from build123d import *

# Parameters (mm, degrees)
F1_R     = 7.008857
F1_R_2   = 6.918989
F1_R_3   = 6.910628
F1_R_4   = 85
F1_R_5   = 7.545233
F2_DEPTH = 3


with BuildPart() as f2:
    # F1 (on Top) → F2 (new body)
    with BuildSketch(Plane.XY):
        with BuildLine():
            ThreePointArc((133.07327, 178.290789), (197.066851, 100.910925), (219.991151, 3.14949))
            ThreePointArc((219.991151, 3.14949), (197.066851, -94.611945), (133.07327, -171.991809))
            Line((133.07327, -171.991809), (156.635002, -171.991809))
            ThreePointArc((156.635002, -171.991809), (214.509219, -92.785593), (234.991151, 3.14949))
            ThreePointArc((234.991151, 3.14949), (214.509219, 99.084573), (156.635002, 178.290789))
            Line((156.635002, 178.290789), (133.07327, 178.290789))
        make_face()
        with BuildLine():
            ThreePointArc((-132.922132, -171.991809), (-219.840013, 3.14949), (-132.922132, 178.290789))
            Line((-132.922132, 178.290789), (-156.483864, 178.290789))
            ThreePointArc((-156.483864, 178.290789), (-234.840013, 3.14949), (-156.483864, -171.991809))
            Line((-156.483864, -171.991809), (-132.922132, -171.991809))
        make_face()
        with BuildLine():
            ThreePointArc((133.07327, -171.991809), (197.066851, -94.611945), (219.991151, 3.14949))
            ThreePointArc((219.991151, 3.14949), (197.066851, 100.910925), (133.07327, 178.290789))
            Line((133.07327, 178.290789), (-132.922132, 178.290789))
            ThreePointArc((-132.922132, 178.290789), (-219.840013, 3.14949), (-132.922132, -171.991809))
            Line((-132.922132, -171.991809), (133.07327, -171.991809))
        make_face()
        with Locations((-155.586369, -87.818066)):
            Circle(F1_R, mode=Mode.SUBTRACT)
        with Locations((141.81215, -93.474258)):
            Circle(F1_R_2, mode=Mode.SUBTRACT)
        with Locations((-140.995276, 99.463245)):
            Circle(F1_R_3, mode=Mode.SUBTRACT)
        with Locations((0.075569, 3.14949)):
            Circle(F1_R_4, mode=Mode.SUBTRACT)
        with Locations((142.390701, 98.258993)):
            Circle(F1_R_5, mode=Mode.SUBTRACT)
    extrude(amount=F2_DEPTH)


solid = f2.part
The model under review builds one solid part; all positions refer to its coordinate system, in mm. Round coordinates to 2 decimals unless told otherwise and drop trailing zeros. Order: outer loops, then holes, each group sorted by start corner. A loop starts at its lowest first (then second) coordinate and runs counter-clockwise, first axis right, second up. Notation, with made-up numbers: (42.25, -37) -> (46.25, -37) arc R28 ccw to (46.25, -14) -> close; hole circle Ø5 at (-29.75, 44.25). An arc over 180 degrees is marked (long way). Return JSON: item names as keys, results as strings.
1. The part is to be moulded in two halves that separate along Y. For faces 1 (the face through (49, 83, 0)), 2 (the face through (-234.824, 5.917, 1.479)), 3 (the face through (-149.11, -90.5, 1.48)), say which applies: +Y half, -Y half, draft (parallel to the pull), parting line (faces both ways), or undercut.
Answer block:
{"face 1": "draft", "face 2": "parting line", "face 3": "undercut"}
2. For L1, parallel to Y at x = 145.5, z = 1.3; L2, parallel to X at y = 94, z = 2.3; L3, parallel to Y at x = -6.5, z = 1.2, list the stretches that pass through material, from the lowest coordinate up. Write a range as [from, to].
Answer block:
{"L1": "y = [-171.99, -99.33], [-87.62, 91.38], [105.13, 178.29]", "L2": "x = [-216.56, -145.23], [-136.76, 136.16], [148.62, 216.71]", "L3": "y = [-171.99, -81.6], [87.89, 178.29]"}
3. Take a section at D-D (y = -147). Write out the cut boundary in (x, z), then the cut area to 3 significant figures.
Answer block:
{"outline": "(-180.59, 0) -> (180.74, 0) -> (180.74, 3) -> (-180.59, 3) -> close", "area": "1,080 mm²"}
4. Take a section at B-B (x = -73.5). Write out the cut boundary in (y, z), then the cut area to 3 significant figures.
Answer block:
{"outline": "(-171.99, 0) -> (-39.41, 0) -> (-39.41, 3) -> (-171.99, 3) -> close; (45.71, 0) -> (178.29, 0) -> (178.29, 3) -> (45.71, 3) -> close", "area": "795 mm²"}
5. Take a section at C-C (z = 1.25). Write out the cut boundary in (x, y) (1 decimal), then the cut area to 3 significant figures.
Answer block:
{"outline": "(-156.5, -172) -> (156.6, -172) arc R234.9 ccw to (235, 3.1) arc R234.9 ccw to (156.6, 178.3) -> (-156.5, 178.3) arc R234.9 ccw to start; hole circle Ø14 at (-155.6, -87.8); hole circle Ø13.8 at (-141, 99.5); hole circle Ø170 at (0.1, 3.1); hole circle Ø15.1 at (142.4, 98.3); hole circle Ø13.8 at (141.8, -93.5)", "area": "124,000 mm²"}
6. Take a section at A-A (y = -22). Write out the cut boundary in (x, z).
Answer block:
{"outline": "(-233.49, 0) -> (-81.12, 0) -> (-81.12, 3) -> (-233.49, 3) -> close; (81.27, 0) -> (233.64, 0) -> (233.64, 3) -> (81.27, 3) -> close"}
